from build123d import *

# Parameters (mm, degrees)
SKETCH003_R     = 4.9
PAD002_DEPTH    = 2
SKETCH004_R     = 5.5
PAD003_DEPTH    = 1
CHAMFER005_SIZE = 0.5


with BuildPart() as part:
    # Sketch003 → Pad002 (new body)
    with BuildSketch(Plane.XZ):
        with Locations((-27.765049, 49.769871)):
            Circle(SKETCH003_R)
    extrude(amount=PAD002_DEPTH)

    # Sketch004 (on Face2 of Pad002) → Pad003 (join)
    with BuildSketch(Plane(origin=(0, 0, 0), x_dir=(1, 0, 0), z_dir=(0, 1, 0))):
        with Locations((-27.765049, -49.769871)):
            Circle(SKETCH004_R)
    extrude(amount=PAD003_DEPTH)

    # Chamfer005
    chamfer005_edges = [part.edges().sort_by_distance(p)[0] for p in [
        (-33.265049, 0, 49.769871),
    ]]
    chamfer(chamfer005_edges, length=CHAMFER005_SIZE)


with BuildPart() as part_1:
    # Body001 placement: moved
    add(part.part.moved(Location((1.3, -51.8, -37.8))))


solid = part_1.part
Verification items for the finished model (mm, model axes). A direction names the side the tool comes from. Give positions to 0.01 mm unless a question says otherwise; leave off trailing zeros. Loops run counter-clockwise (first coordinate to the right, second up) from the corner with the lowest first, then second, coordinate; pieces in that order, holes last.
1. Cross-section at A-A on y = -51.65. Record the cut outline in (x, z), and give its area (3 significant figures).
Derived:
outline: circle Ø10.3 at (-26.47, 11.97)
area: 83.3 mm2
2. Go/stop test with flat-tipped pins: P1, Ø1.5, axis at x = -24.5, y = -52.5, coming from the +Z side; P2, Ø1.5, axis at x = -23.5, y = -51, coming from the -Z side; P3, Ø1, axis at y = -51, z = 11.5, coming from the +X side. Record where each tip stops, or that it passes through.
Derived:
P1: stops at z = 16.72
P2: stops at z = 6.94
P3: stops at x = -20.97
3. Material ranges on probe 1 along Y at (x, z) = (-29, 16.25); probe 2 along Z at (x, y) = (-28.5, -52.3); probe 3 along Z at (x, y) = (-30, -53.1), recorded low to high.
Derived:
probe 1: y = -51.8 to -50.8
probe 2: z = 7.51 to 16.43
probe 3: z = 8.58 to 15.36
4. Cross-section at B-B on y = -53.45. Record the cut outline in (x, z).
Derived:
outline: circle Ø9.8 at (-26.47, 11.97)
5. Tool access check on faces 1 (the cylindrical face through (-21.94, -52.79, 10.09)), 2 (the flat face through (-27, -53.8, 12)). Record the directions out of +Z, -Z, +X, -X, +Y, -Y that give a thin tool (end or side, any length) a straight path to the whole face; none if there is none.
Derived:
face 1: -Y
face 2: +Z, -Z, +X, -X, -Y
